Autodesk Inventor part; units mm, degrees
ref_plane "YZ Plane" through (0, 0, 0) normal (1, 0, 0) x (0, 1, 0)
ref_plane "XZ Plane" through (0, 0, 0) normal (0, 1, 0) x (-1, 0, 0)
ref_plane "XY Plane" through (0, 0, 0) normal (0, 0, 1) x (1, 0, 0)
sketch "Sketch1" plane through (0, 0, 0) normal (1, 0, 0) x (0, 1, 0)
  line L0 (-184, -384) -> (184, -384)
  line L1 (184, -384) -> (184, 384)
  line L2 (184, 384) -> (-184, 384)
  line L3 (-184, 384) -> (-184, -384)
  line L4 (-184, -384) -> (184, 384) construction
  line L5 (184, -384) -> (-184, 384) construction
  line L6 (159, 350) -> (84, 350)
  line L7 (84, 350) -> (84, 150)
  line L8 (84, 150) -> (159, 150)
  line L9 (159, 150) -> (159, 350)
  line L10 (159, -100) -> (159, 100)
  line L11 (159, 100) -> (84, 100)
  line L12 (84, 100) -> (84, -100)
  line L13 (84, -100) -> (159, -100)
  line L14 (159, -350) -> (159, -150)
  line L15 (159, -150) -> (84, -150)
  line L16 (84, -150) -> (84, -350)
  line L17 (84, -350) -> (159, -350)
  circle A0 centre (-75, 0) radius 25
  point P0 (0, 0)
  dimension "d0" = 768
  dimension "d1" = 368
  dimension "d2" = 200
  dimension "d3" = 75
  dimension "d4" = 34
  dimension "d5" = 25
  dimension "d8" = 250
  dimension "d17" = 75
  dimension "d18" = 50
extrude "Extrusion1" add sketch "Sketch1" along normal mid plane 3
properties part number "Posterior" material "Acrylic"
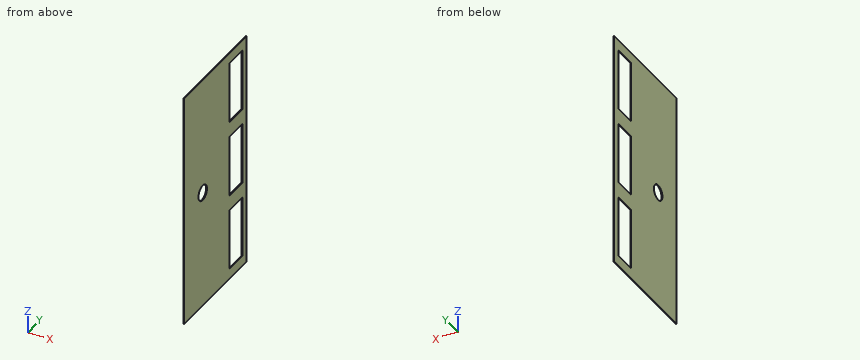
For this review, take the finished solid that the model builds, in its own axes (mm). Round coordinates to 2 decimals unless told otherwise and drop trailing zeros. Loops run counter-clockwise (first coordinate to the right, second up) from the corner with the lowest first, then second, coordinate; pieces in that order, holes last. Notation, with made-up numbers: (47.25, 77.25) - (101.25, 77.25) arc R33 ccw to (101.25, 116.25) - close; hole circle Ø6 at (72, 10.25). An arc over 180 degrees is marked (long way). Answer as CSV lines item,"result".
(1) Consider section D-D on z = -300. Give the boundary of the cut face in (x, y), then the cut area to 3 significant figures.
Checked values:
outline,"(-1.5, -184) - (1.5, -184) - (1.5, 84) - (-1.5, 84) - close; (-1.5, 159) - (1.5, 159) - (1.5, 184) - (-1.5, 184) - close"
area,"879 mm2"
(2) Consider section B-B on x = 1.05. Give the boundary of the cut face in (y, z).
Checked values:
outline,"(-184, -384) - (184, -384) - (184, 384) - (-184, 384) - close; hole circle Ø50 at (-75, 0); hole (84, -350) - (159, -350) - (159, -150) - (84, -150) - close; hole (84, -100) - (159, -100) - (159, 100) - (84, 100) - close; hole (84, 150) - (159, 150) - (159, 350) - (84, 350) - close"
(3) Wall thickness on line 1 (Z direction, x = 0.85, y = 135); line 2 (Y direction, x = 1.2, z = -189); line 3 (Z direction, x = 0.85, y = -75): over which ranges is each line inside the solid? List them lowest first.
Checked values:
line 1,"z = -384 to -350, -150 to -100, 100 to 150, 350 to 384"
line 2,"y = -184 to 84, 159 to 184"
line 3,"z = -384 to -25, 25 to 384"
(4) Consider section A-A on y = -75. Give the boundary of the cut face in (x, z).
Checked values:
outline,"(-1.5, -384) - (1.5, -384) - (1.5, -25) - (-1.5, -25) - close; (-1.5, 25) - (1.5, 25) - (1.5, 384) - (-1.5, 384) - close"
(5) Consider section C-C on z = 0. Give the boundary of the cut face in (x, y).
Checked values:
outline,"(-1.5, -184) - (1.5, -184) - (1.5, -100) - (-1.5, -100) - close; (-1.5, -50) - (1.5, -50) - (1.5, 84) - (-1.5, 84) - close; (-1.5, 159) - (1.5, 159) - (1.5, 184) - (-1.5, 184) - close"
